Solid Edge part; units mm, degrees
sketch "Sketch1" plane through (0, 0, 0) normal (0, 0, 1) x (1, 0, 0)
  line L0 (-4, 3.6) -> (4, 3.6)
  line L1 (-4, -3.6) -> (4, -3.6)
  arc A0 (-4, -3.6) -> (-4, 3.6) centre (-4, 0) cw
  arc A1 (4, 3.6) -> (4, -3.6) centre (4, 0) cw
  line L2 (-1.7373, 2.8) -> (1.7373, 2.8)
  arc A2 (1.7373, -2.8) -> (1.7373, 2.8) centre (4, 0) cw
  line L3 (-1.7373, -2.8) -> (1.7373, -2.8)
  arc A3 (-0.5143, -0.9) -> (-1.7373, -2.8) centre (-4, 0) cw
  line L4 (-0.5143, -0.9) -> (-3.1, -0.9)
  line L5 (-3.1, -2.2249) -> (-3.1, -0.9)
  line L6 (-4.9, -0.9) -> (-4.9, -2.2249)
  line L7 (-4.9, -0.9) -> (-6.2249, -0.9)
  arc A4 (-6.2249, -0.9) -> (-6.2249, 0.9) centre (-4, 0) cw
  line L8 (-6.2249, 0.9) -> (-4.9, 0.9)
  line L9 (-4.9, 2.2249) -> (-4.9, 0.9)
  arc A5 (-4.9, 2.2249) -> (-3.1, 2.2249) centre (-4, 0) cw
  line L10 (-3.1, 0.9) -> (-3.1, 2.2249)
  line L11 (-3.1, 0.9) -> (-0.5143, 0.9)
  arc A6 (-1.7373, 2.8) -> (-0.5143, 0.9) centre (-4, 0) cw
  arc A7 (-3.1, -2.2249) -> (-4.9, -2.2249) centre (-4, 0) cw
extrude "Protrusion1" add sketch "Sketch1" along normal blind 8
fillet "Round_1" radius 0.5 10 edges at (-1.7373, 2.8, 4) (-0.5143, 0.9, 4) (1.7373, 2.8, 4) (-0.5143, -0.9, 4) (-1.7373, -2.8, 4) (-4.9, -0.9, 4) (-4.9, 0.9, 4) (-3.1, 0.9, 4) (-3.1, -0.9, 4) (1.7373, -2.8, 4)
fillet "Round_2" radius 0.1 6 edges at (-4.9, 2.2249, 4) (-3.1, 2.2249, 4) (-6.2249, -0.9, 4) (-6.2249, 0.9, 4) (-4.9, -2.2249, 4) (-3.1, -2.2249, 4)
sketch "Sketch2" plane through (0, 0, 0) normal (0, -1, 0) x (1, 0, 0)
  line L0 (7.1, 0) -> (4, 0)
  line L1 (7.1, 0.8) -> (7.1, 0)
  line L2 (6.4, 0.8) -> (7.1, 0.8)
  line L3 (6.4, 7.2) -> (6.4, 0.8)
  line L4 (7.1, 7.2) -> (6.4, 7.2)
  line L5 (7.1, 8) -> (7.1, 7.2)
  line L6 (4, 8) -> (7.1, 8)
revolve "RevolvedCutout1" cut sketch "Sketch2" angle 360 about axis through (4, 0, 0) along (0, 0, 1)
Model file for the job. Use its own axes, mm. A direction names the side the tool comes from. Give positions to 0.01 mm unless a question says otherwise; leave off trailing zeros. Loops run counter-clockwise (first coordinate to the right, second up) from the corner with the lowest first, then second, coordinate; pieces in that order, holes last. Notation, with made-up numbers: (4.5, 67.5) -> (10.5, 67.5) arc R27 ccw to (10.5, 86.5) -> close; hole circle Ø6 at (81.25, 6). An arc over 180 degrees is marked (long way). Use a Markdown table: item, result. Add a question column.
(1) Slice it at C-C on z = 2. Give the number of separate pieces and of enclosed holes in the cut face, and give its area (3 significant figures).
(2) Slice it at A-A on y = 0. List the corners of the cut face in (x, z).
(3) Tool access for faces 1 (the cylindrical face through (-6.4, 0, 3.9)), 2 (the flat face through (6, -2, 7.2)), 3 (the cylindrical face through (7.6, 0.1, 3.9)): list every direction of +Z, -Z, +X, -X, +Y, -Y with a clear straight run to the whole face (end or side of a thin tool).
(4) Wall check: line 1 along Y through (x, z) = (4, 5.5); line 2 along X through (y, z) = (1.5, 0.5); line 3 along Y through (x, z) = (-2.5, 6). Give the ranges that are in metal, low to high.
(5) Mould opens along Y. For faces 4 (the flat face through (0, 3.6, 4)), 5 (the cylindrical face through (1.54, 1.886, 0.394)), 6 (the flat face through (0, -3.6, 4)), 7 (the cylindrical face through (-4, -2.4, 3.9)) say: +Y half, -Y half, draft (parallel to the pull), parting line (faces both ways), or undercut.
(6) Slice it at B-B on x = -5.75. List the corners of the cut face in (y, z).
(7) Drop flat-ended pins along their axis: pin 1 Ø2 at (y, z) = (2.5, 5.5) entering from +X; pin 2 Ø0.8 at (y, z) = (-1.5, 3) entering from -X. Give the stop position or say it passes through.
(8) Slice it at D-D on x = 3. List the corners of the cut face in (y, z).
Filled sheet:
| question | item | result |
|---|---|---|
| 1 | separate pieces | 1 |
| 1 | enclosed holes | 2 |
| 1 | area | 55.9 mm2 |
| 2 | outline | (-7.6, 0) -> (-6.4, 0) -> (-6.4, 8) -> (-7.6, 8) -> close; (0.4, 0) -> (0.9, 0) -> (0.9, 0.8) -> (1.6, 0.8) -> (1.6, 7.2) -> (0.9, 7.2) -> (0.9, 8) -> (0.4, 8) -> close; (6.4, 0.8) -> (7.1, 0.8) -> (7.1, 0) -> (7.6, 0) -> (7.6, 8) -> (7.1, 8) -> (7.1, 7.2) -> (6.4, 7.2) -> close |
| 3 | face 1 | +Z, -Z |
| 3 | face 2 | +Z |
| 3 | face 3 | +Z, -Z, +X |
| 4 | line 1 | -3.6 to -2.4, 2.4 to 3.6 |
| 4 | line 2 | -7.27 to -4.9, -3.1 to -0.74, 0.73 to 1.29, 6.71 to 7.27 |
| 4 | line 3 | -3.6 to -0.9, 0.9 to 3.6 |
| 5 | face 4 | +Y half |
| 5 | face 5 | undercut |
| 5 | face 6 | -Y half |
| 5 | face 7 | undercut |
| 6 | outline | (-3.15, 0) -> (-0.9, 0) -> (-0.9, 8) -> (-3.15, 8) -> close; (0.9, 0) -> (3.15, 0) -> (3.15, 8) -> (0.9, 8) -> close |
| 7 | pin 1 | x = 7.27 |
| 7 | pin 2 | x = -7.43 |
| 8 | outline | (-3.6, 0) -> (-2.93, 0) -> (-2.93, 0.8) -> (-2.18, 0.8) -> (-2.18, 7.2) -> (-2.93, 7.2) -> (-2.93, 8) -> (-3.6, 8) -> close; (2.18, 0.8) -> (2.93, 0.8) -> (2.93, 0) -> (3.6, 0) -> (3.6, 8) -> (2.93, 8) -> (2.93, 7.2) -> (2.18, 7.2) -> close |
